Here's how the part is built. I have some questions about the finished solid (model axes, mm). A direction names the side the tool comes from. Give positions to 0.01 mm unless a question says otherwise; leave off trailing zeros. Loops run counter-clockwise (first coordinate to the right, second up) from the corner with the lowest first, then second, coordinate; pieces in that order, holes last. Notation, with made-up numbers: M 10.25,-21.75 L 69.25,-21.75 A11 cw 69.25,-11.75 Z; hole C 84,53.25 d3. An arc over 180 degrees is marked long. Write item = value, one per line. Start each with the question number.
```python
from build123d import *

# Parameters (mm, degrees)
F0_R     = 3.175
F1_DEPTH = 25.4
F2_R     = 4.7625
F3_DEPTH = 6.35
F5_DEPTH = 5.08


with BuildPart() as f1:
    # F0 (on Front) → F1 (new body)
    with BuildSketch(Plane.XZ):
        Circle(F0_R)
    extrude(amount=F1_DEPTH)

    # F2 (on face) → F3 (join)
    with BuildSketch(Plane.XZ.offset(25.4)):
        Circle(F2_R)
    extrude(amount=F3_DEPTH)

    # F4 (on face) → F5 (cut)
    with BuildSketch(Plane.XZ.offset(31.75)):
        Polygon((-3.119147, 0.592914), (-2.073052, -2.404803), (1.046095, -2.997718), (3.119147, -0.592914), (2.073052, 2.404803), (-1.046095, 2.997718), align=None)
    extrude(amount=-F5_DEPTH, mode=Mode.SUBTRACT)


solid = f1.part
```
Q1. If we section it at A-A, the plane y = -27.5: List the corners of the cut face in (x, z) for me (1 decimal), then the cut area to 3 significant figures.
Q2. Will these pins go through, and if not, where does the flat tip stop? pin 1 (4 mm diameter, centred on x = -3.5, y = -25.5, fed in from +Z); pin 2 (3 mm diameter, centred on y = -7.5, z = -1, fed in from +X) (3 decimals); pin 3 (4 mm diameter, centred on x = -2, y = -11, fed in from +Z) (3 decimals).
Q3. If we section it at D-D, the plane y = -15: List the corners of the cut face in (x, z) for me (3 decimals), then the cut area to 3 significant figures.
Q4. On a 3-axis mill with a long thin cutter (end or side, diameter ignored), from which of +Z, -Z, +X, -X, +Y, -Y can I reach the whole of each face in a straight line? I mean faces 4 (the flat face through (0, -31.75, -3)), 5 (the flat face through (-0.535, -29.246, -2.697)). Say none if no direction works.
Q5. If I drill on line 1 along Y through (x, z) = (-1.75, -2.25); line 2 along Y through (x, z) = (-0.75, 3.75); line 3 along Z through (x, y) = (3.5, -29), over which ranges is the centre line in solid material (lowest first)?
Q6. We'd pull the mould along X, two halves only. Please class faces 1 (the flat face through (2.6, -29.2, 0.9)), 2 (the cylindrical face through (-0.69, -12.52, -3.1)), 3 (the flat face through (0, 0, 0)): pulls with the +X half, pulls with the -X half, needs draft (parallel to the pull), parting line crosses it, or undercut.
Resolved:
q1.outline = C 0,0 d9.5; hole M -3.1,0.6 L -2.1,-2.4 L 1,-3 L 3.1,-0.6 L 2.1,2.4 L -1,3 Z
q1.area = 45.1 mm²
q2.pin_1 = 4.52
q2.pin_2 = 3.175
q2.pin_3 = 3.175
q3.outline = C 0,0 d6.35
q3.area = 31.7 mm²
q4.face_4 = +Z, -Z, +X, -X, -Y
q4.face_5 = -Y
q5.line_1 = -26.67 to 0
q5.line_2 = -31.75 to -25.4
q5.line_3 = -3.23 to 3.23
q6.face_1 = undercut
q6.face_2 = parting line crosses it
q6.face_3 = needs draft
